Part model, mm, in its own coordinate system. Give positions to 0.01 mm unless a question says otherwise; leave off trailing zeros. Order: outer loops, then holes, each group sorted by start corner. A loop starts at its lowest first (then second) coordinate and runs counter-clockwise, first axis right, second up. Notation, with made-up numbers: M 83.25,62 L 91.25,62 A17 ccw 91.25,87 Z; hole C 72,-34.5 d7. An arc over 180 degrees is marked long. Write each question's results on one line, items separated by ' | '. Start each with the question number.
Autodesk Inventor part; units mm, degrees
ref_plane "YZ Plane" through (0, 0, 0) normal (1, 0, 0) x (0, 1, 0)
ref_plane "XZ Plane" through (0, 0, 0) normal (0, 1, 0) x (-1, 0, 0)
ref_plane "XY Plane" through (0, 0, 0) normal (0, 0, 1) x (1, 0, 0)
sketch "Sketch1" plane through (0, 0, 0) normal (0, 1, 0) x (-1, 0, 0)
  circle A0 centre (0, 0) radius 25
  dimension "d0" = 50
extrude "Extrusion1" add sketch "Sketch1" along normal blind 20
draft "FaceDraft1" angle 8 pull direction (0, 1, 0) faces at (-24.9189, 13.3333, -2.0117) fixed edges at (25, 20, 0)
sketch "Sketch2" plane through (0, 20, 0) normal (0, 1, 0) x (1, 0, 0)
  point P0 (0, 0)
  point P1 (0, 0)
hole "Hole1" at (0, 20, 0) direction (0, -1, 0) diameter 3 end through all
properties part number "shoulder_base"
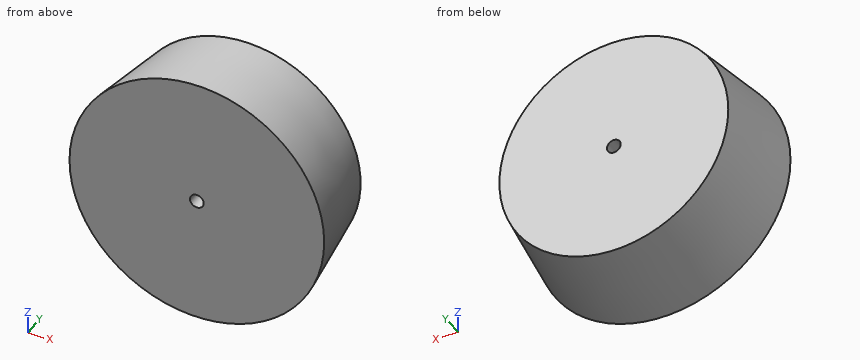
(1) Probe L1, parallel to Z at x = 0, y = 9.5; L2, parallel to Z at x = 0, y = 10.5; L3, parallel to X at y = 14, z = 0. List the from-to ranges inside material, lowest first.
(2) Saw through at D-D on y = 10. Give the cut face in (x, z), plus the area to 3 significant figures.
(3) Saw through at C-C on y = 4.25. Give the cut face in (x, z).
(4) Drop flat-ended pins along their axis: P1, Ø6, axis at y = 9, z = 6, coming from the -X side; P2, Ø6, axis at x = -11, y = 13, coming from the +Z side; P3, Ø6, axis at y = 9, z = 13.5, coming from the +X side. Give the stop position or say it passes through.
(5) Saw through at A-A on x = 0. Give the cut face in (y, z).
(6) Saw through at B-B on z = 0. Give the cut face in (x, y).
Taken from the geometry:
1) L1: z = -26.48 to -1.5, 1.5 to 26.48 | L2: z = -26.34 to -1.5, 1.5 to 26.34 | L3: x = -25.84 to -1.5, 1.5 to 25.84
2) outline: C 0,0 d52.81; hole C 0,0 d3 | area: 2,180 mm²
3) outline: C 0,0 d54.43; hole C 0,0 d3
4) P1: stops at x = -26.56 | P2: stops at z = 24.82 | P3: stops at x = 24.46
5) outline: M 0,-27.81 L 20,-25 L 20,-1.5 L 0,-1.5 Z; M 0,1.5 L 20,1.5 L 20,25 L 0,27.81 Z
6) outline: M -27.81,0 L -1.5,0 L -1.5,20 L -25,20 Z; M 1.5,0 L 27.81,0 L 25,20 L 1.5,20 Z
